Design review of the part built by this model. Coordinates are the model's own, in mm. Face numbers are marked on the shaded views. Coordinates: 2 decimals unless noted, no trailing zeros. Write each loop counter-clockwise with the first axis right and the second up, starting at its lowest first coordinate (ties: lowest second). Pieces come first, ordered by that corner, then holes. Notation, with made-up numbers: M 57,50 L 109,50 A20 ccw 109,67 Z; hole C -14.75,80.25 d2. An arc over 180 degrees is marked long. Write item = value, one per line.
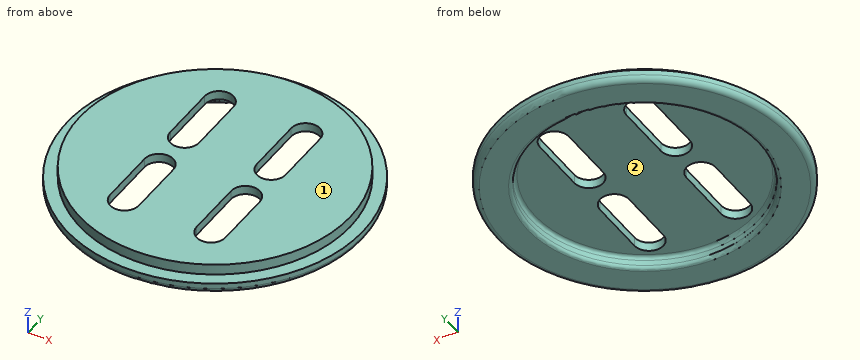
```python
from build123d import *

# Parameters (mm, degrees)
SKETCH1_R           = 41
BOSS_EXTRUDE1_DEPTH = 3
SKETCH2_R           = 37.5
BOSS_EXTRUDE4_DEPTH = 3
SKETCH5_R           = 31.5
CUT_EXTRUDE3_DEPTH  = 3.5
CUT_EXTRUDE6_DEPTH  = 3
FILLET3_R           = 1
FILLET4_R           = 1.5
FILLET5_R           = 1


with BuildPart() as part:
    # Sketch1 → Boss-Extrude1 (new body)
    with BuildSketch(Plane.XY):
        Circle(SKETCH1_R)
    extrude(amount=BOSS_EXTRUDE1_DEPTH)

    # Sketch2 → Boss-Extrude4 (add)
    with BuildSketch(Plane.XY.offset(3)):
        Circle(SKETCH2_R)
    extrude(amount=BOSS_EXTRUDE4_DEPTH)

    # Sketch5 → Cut-Extrude3 (cut)
    with BuildSketch(Plane(origin=(0, 0, 0), x_dir=(-1, 0, 0), z_dir=(0, 0, -1))):
        Circle(SKETCH5_R)
    extrude(amount=-CUT_EXTRUDE3_DEPTH, mode=Mode.SUBTRACT)

    # Sketch6 → Cut-Extrude6 (cut)
    with BuildSketch(Plane(origin=(0, 0, 3.5), x_dir=(-1, 0, 0), z_dir=(0, 0, -1))):
        with BuildLine():
            Line((-16, 6), (-16, 22))
            ThreePointArc((-16, 22), (-12, 26), (-8, 22))
            Line((-8, 22), (-8, 6))
            ThreePointArc((-8, 6), (-12, 2), (-16, 6))
        make_face()
        with BuildLine():
            Line((16, 6), (16, 22))
            ThreePointArc((16, 22), (12, 26), (8, 22))
            Line((8, 22), (8, 6))
            ThreePointArc((8, 6), (12, 2), (16, 6))
        make_face()
        with BuildLine():
            Line((16, -6), (16, -22))
            ThreePointArc((16, -22), (12, -26), (8, -22))
            Line((8, -22), (8, -6))
            ThreePointArc((8, -6), (12, -2), (16, -6))
        make_face()
        with BuildLine():
            Line((-16, -6), (-16, -22))
            ThreePointArc((-16, -22), (-12, -26), (-8, -22))
            Line((-8, -22), (-8, -6))
            ThreePointArc((-8, -6), (-12, -2), (-16, -6))
        make_face()
    extrude(amount=-CUT_EXTRUDE6_DEPTH, mode=Mode.SUBTRACT)

    # Fillet3
    fillet3_edges = [part.edges().sort_by_distance(p)[0] for p in [
        (31.5, 0, 0),
    ]]
    fillet(fillet3_edges, radius=FILLET3_R)

    # Fillet4
    fillet4_edges = [part.edges().sort_by_distance(p)[0] for p in [
        (-41, 0, 0),
    ]]
    fillet(fillet4_edges, radius=FILLET4_R)

    # Fillet5
    fillet5_edges = [part.edges().sort_by_distance(p)[0] for p in [
        (31.5, 0, 3.5),
    ]]
    fillet(fillet5_edges, radius=FILLET5_R)


solid = part.part
```
Q1. For P1, Ø1.2, axis at y = 13, z = 4.5, coming from the +X side; P2, Ø3, axis at y = -16.5, z = 5, coming from the +X side; P3, Ø6, axis at x = -12.5, y = 23, coming from the -Z side, all flat-tipped, find the tip position at first contact; note any pin that passes through.
Check result:
P1 = 35.39
P2 = 34.37
P3 = 3.5
Q2. Wall thickness on line 1 (X direction, y = -23, z = 4.8); line 2 (X direction, y = -14, z = 5.3); line 3 (Y direction, x = 0, z = 1.6): over which ranges is each line inside the solid? List them lowest first.
Check result:
line_1 = -29.62 to -15.87, -8.13 to 8.13, 15.87 to 29.62
line_2 = -34.79 to -16, -8 to 8, 16 to 34.79
line_3 = -41 to -31.5, 31.5 to 41
Q3. Consider section A-A, the plane z = 4.6. State the section outline as (x, y) points.
Check result:
outline = C 0,0 d75; hole M -16,-22 A4 ccw -8,-22 L -8,-6 A4 ccw -16,-6 Z; hole M -16,6 A4 ccw -8,6 L -8,22 A4 ccw -16,22 Z; hole M 8,-22 A4 ccw 16,-22 L 16,-6 A4 ccw 8,-6 Z; hole M 8,6 A4 ccw 16,6 L 16,22 A4 ccw 8,22 Z
Q4. The part is to be moulded in two halves that separate along Y. For the marked faces 1 and 2, say which applies: +Y half, -Y half, draft (parallel to the pull), parting line (faces both ways), or undercut.
Check result:
face_1 = draft
face_2 = undercut
Q5. Consider section B-B, the plane x = 0. State the section outline as (y, z) points, and give its area (3 significant figures).
Check result:
outline = M -41,1.5 A1.5 ccw -39.5,0 L -32.5,0 A1 ccw -31.5,1 L -31.5,2.5 A1 cw -30.5,3.5 L 30.5,3.5 A1 cw 31.5,2.5 L 31.5,1 A1 ccw 32.5,0 L 39.5,0 A1.5 ccw 41,1.5 L 41,3 L 37.5,3 L 37.5,6 L -37.5,6 L -37.5,3 L -41,3 Z
area = 250 mm²
Q6. Consider section C-C, the plane y = -13. State how many separate pieces and enclosed holes the cut face has, and give its area (3 significant figures).
Check result:
separate_pieces = 3
enclosed_holes = 0
area = 202 mm²
